from build123d import *

# Parameters (mm, degrees)
EXTRUSION1_DEPTH        = 3
ESQUISSE4_R             = 5
ENL_V_MAT_EXTRU_3_DEPTH = 16
ESQUISSE8_R             = 3
ENL_V_MAT_EXTRU_5_DEPTH = 8
ESQUISSE9_R             = 1.5
ENL_V_MAT_EXTRU_6_DEPTH = 10
ESQUISSE11_W            = 10
ESQUISSE11_H            = 5
ENL_V_MAT_EXTRU_9_DEPTH = 0.0001
EXTRUSION2_DEPTH        = 2
ESQUISSE5_R             = 1.5
ENL_V_MAT_EXTRU_4_DEPTH = 25.792218749
ESQUISSE3_R             = 5
ENL_V_MAT_EXTRU_2_DEPTH = 16


with BuildPart() as part:
    # Esquisse1 → Extrusion1 (new body)
    with BuildSketch(Plane.XY):
        Polygon((0, 0), (-120, 0), (-120, -150), (-70, -200), (-50, -200), (0, -150), align=None)
    extrude(amount=EXTRUSION1_DEPTH)

    # Esquisse4 → Enlèv. mat.-Extru.3 (cut)
    with BuildSketch(Plane(origin=(0, 0, 0), x_dir=(-1, 0, 0), z_dir=(0, 0, -1))):
        with Locations((60, -10)):
            Circle(ESQUISSE4_R)
        with Locations((10, -85)):
            Circle(ESQUISSE4_R)
        with Locations((110, -85)):
            Circle(ESQUISSE4_R)
    extrude(amount=-ENL_V_MAT_EXTRU_3_DEPTH, mode=Mode.SUBTRACT)

    # Esquisse8 → Enlèv. mat.-Extru.5 (cut)
    with BuildSketch(Plane(origin=(0, 0, 0), x_dir=(-1, 0, 0), z_dir=(0, 0, -1))):
        with Locations((52.5, -23)):
            Circle(ESQUISSE8_R)
        with Locations((42.5, -23)):
            Circle(ESQUISSE8_R)
        with Locations((67.5, -23)):
            Circle(ESQUISSE8_R)
        with Locations((77.5, -23)):
            Circle(ESQUISSE8_R)
    extrude(amount=-ENL_V_MAT_EXTRU_5_DEPTH, mode=Mode.SUBTRACT)

    # Esquisse9 → Enlèv. mat.-Extru.6 (cut)
    with BuildSketch(Plane(origin=(0, 0, 0), x_dir=(-1, 0, 0), z_dir=(0, 0, -1))):
        with Locations((60, -143)):
            Circle(ESQUISSE9_R)
        with Locations((60, -188)):
            Circle(ESQUISSE9_R)
    extrude(amount=-ENL_V_MAT_EXTRU_6_DEPTH, mode=Mode.SUBTRACT)

    # Esquisse11 → Enlèv. mat.-Extru.9 (cut)
    with BuildSketch(Plane.XY.offset(3)):
        with Locations((-115, -23)):
            Rectangle(ESQUISSE11_W, ESQUISSE11_H)
        with Locations((-5, -23)):
            Rectangle(ESQUISSE11_W, ESQUISSE11_H)
    extrude(amount=-ENL_V_MAT_EXTRU_9_DEPTH, mode=Mode.SUBTRACT)

    # Esquisse12 → Extrusion2 (add)
    with BuildSketch(Plane(origin=(0, 0, 0), x_dir=(-1, 0, 0), z_dir=(0, 0, -1))):
        Polygon((30, -133.99467083), (30, -137), (31.859648796, -137), (31.859648796, -139), (28, -139), (28, -133.99467083), align=None)
    extrude(amount=EXTRUSION2_DEPTH)

    # Esquisse5 → Enlèv. mat.-Extru.4 (cut)
    with BuildSketch(Plane.XY):
        with Locations(Location((-77, -68, 0), (0, 0, 180))):
            Circle(ESQUISSE5_R)
        with Locations(Location((-43, -68, 0), (0, 0, 180))):
            Circle(ESQUISSE5_R)
        with Locations(Location((-43, -92, 0), (0, 0, 180))):
            Circle(ESQUISSE5_R)
        with Locations(Location((-77, -92, 0), (0, 0, 180))):
            Circle(ESQUISSE5_R)
    extrude(amount=ENL_V_MAT_EXTRU_4_DEPTH, mode=Mode.SUBTRACT)

    # Esquisse3 → Enlèv. mat.-Extru.2 (cut)
    with BuildSketch(Plane(origin=(0, 0, 0), x_dir=(-1, 0, 0), z_dir=(0, 0, -1))):
        with Locations((60, -58)):
            Circle(ESQUISSE3_R)
    extrude(amount=-ENL_V_MAT_EXTRU_2_DEPTH, mode=Mode.SUBTRACT)


solid = part.part
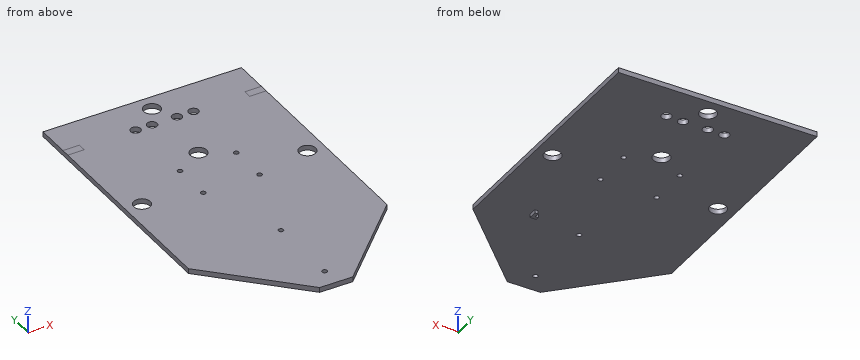
The model under review builds one solid part; all positions refer to its coordinate system, in mm. Coordinates: 2 decimals unless noted, no trailing zeros. Loops run counter-clockwise (first coordinate to the right, second up) from the corner with the lowest first, then second, coordinate; pieces in that order, holes last. Notation, with made-up numbers: M 70.5,-27.75 L 96.5,-27.75 A21 cw 96.5,-12.75 Z; hole C 15,80 d10. An arc over 180 degrees is marked long. Put each result on its own line as item: value. Start each with the question number.
Q1. Add section D-D (y = -152.5). Write out the cut boundary in (x, z).
Q2. Add section C-C (x = -53). Write out the cut boundary in (y, z), and give its area (3 significant figures).
Q3. Add section B-B (z = 0.85). Count the separate pieces of the cut face and the enclosed holes in it, and give its area (3 significant figures).
Q4. Add section A-A (y = -10). Write out the cut boundary in (x, z), and give its area (3 significant figures).
Q5. Wall thickness on line 1 (X direction, y = -68, z = 1.2); line 2 (Y direction, x = -60, z = 2.75); line 3 (Y direction, x = -67.5, z = 2.4): over which ranges is each line inside the solid? List them lowest first.
Q6. Clearance check with flat-ended pins moving along their axes: pin 1 (9.5 mm diameter, centred on x = -67.5, y = -23, fed in from -Z); pin 2 (0.9 mm diameter, centred on x = -31, z = -1.5, fed in from +Y). State where each tip first meets the part, or that it passes through.
Answers:
1. outline: M -117.5,0 L -2.5,0 L -2.5,3 L -117.5,3 Z
2. outline: M -200,0 L -25.96,0 L -25.96,3 L -200,3 Z; M -20.04,0 L 0,0 L 0,3 L -20.04,3 Z
2. area: 582 mm^2
3. separate pieces: 1
3. enclosed holes: 14
3. area: 21,000 mm^2
4. outline: M -120,0 L -65,0 L -65,3 L -120,3 Z; M -55,0 L 0,0 L 0,3 L -55,3 Z
4. area: 330 mm^2
5. line 1: x = -120 to -78.5, -75.5 to -44.5, -41.5 to 0
5. line 2: y = -200 to -189.5, -186.5 to -144.5, -141.5 to -63, -53 to -15, -5 to 0
5. line 3: y = -200 to -26, -20 to 0
6. pin 1: stops at z = 0
6. pin 2: stops at y = -137
